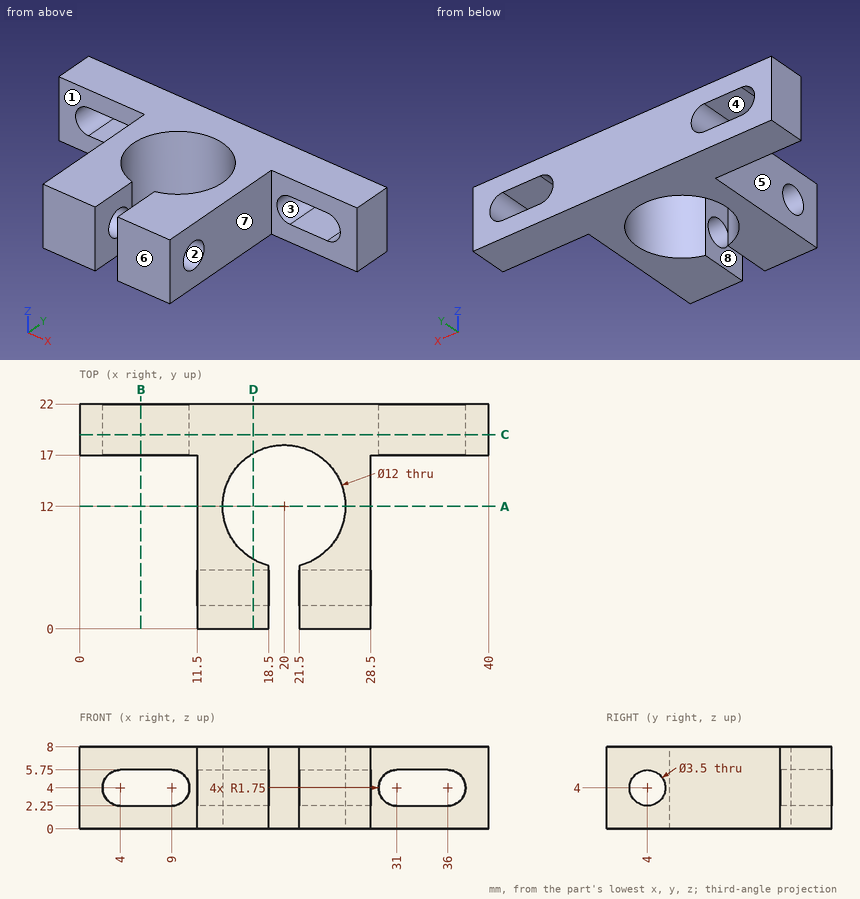
Geometry check sheet. Reference: drawing and pictorial views, mm from the part's lowest x, y, z. A direction names the side the tool comes from. Round coordinates to 2 decimals unless told otherwise and drop trailing zeros. Order: outer loops, then holes, each group sorted by start corner. A loop starts at its lowest first (then second) coordinate and runs counter-clockwise, first axis right, second up. Notation, with made-up numbers: (83.5, 75.25) - (112.5, 75.25) arc R25 ccw to (112.5, 111.25) - close; hole circle Ø2 at (88, -14.75). An arc over 180 degrees is marked (long way). Use a Markdown table: item, result. Add a question column.
1) Section check B-B (x = 6). Record the cut outline in (y, z).
2) Mould release check, pull along Y, two halves, no side actions. Record for the marked faces 1, 2 and 3: released by +Y, released by -Y, zero draft, split by the parting line, or undercut.
3) Thickness scan on line 1 along X through (y, z) = (4.5, 7.5); line 2 along Y through (x, z) = (16, 4.5); line 3 along Y through (x, z) = (25.25, 4). Record the ranges inside material, lowest first.
4) Gauge pin test, flat ends, axial feed: P1, Ø1, axis at x = 17, z = 4, coming from the -Y side; P2, Ø2.5, axis at y = 11.5, z = 4.5, coming from the -X side; P3, Ø4, axis at x = 35.5, z = 3.5, coming from the -Y side; P4, Ø4.5, axis at y = 4, z = 4, coming from the +X side. Record the tip position at first contact, or that the pin passes through.
5) Section check D-D (x = 17). Record the cut outline in (y, z).
6) Section check A-A (y = 12). Record the cut outline in (x, z).
7) Set-up check for the marked faces 4, 5, 6, 7 and 8: record each of +Z, -Z, +X, -X, +Y, -Y from which the full face is reachable in a straight line by a thin tool's end or side.
8) Section check C-C (y = 19). Record the cut outline in (x, z).
Established:
| question | item | result |
|---|---|---|
| 1 | outline | (17, 0) - (22, 0) - (22, 2.25) - (17, 2.25) - close; (17, 5.75) - (22, 5.75) - (22, 8) - (17, 8) - close |
| 2 | face 1 | released by -Y |
| 2 | face 2 | undercut |
| 2 | face 3 | zero draft |
| 3 | line 1 | 11.5 to 18.5, 21.5 to 28.5 |
| 3 | line 2 | 0 to 2.32, 5.68 to 7.53, 16.47 to 22 |
| 3 | line 3 | 0 to 2.25, 5.75 to 9.1, 14.9 to 22 |
| 4 | P1 | y = 0 |
| 4 | P2 | x = 11.5 |
| 4 | P3 | y = 17 |
| 4 | P4 | x = 28.5 |
| 5 | outline | (0, 0) - (6.8, 0) - (6.8, 8) - (0, 8) - close; (17.2, 0) - (22, 0) - (22, 8) - (17.2, 8) - close; hole circle Ø3.5 at (4, 4) |
| 6 | outline | (11.5, 0) - (14, 0) - (14, 8) - (11.5, 8) - close; (26, 0) - (28.5, 0) - (28.5, 8) - (26, 8) - close |
| 7 | face 4 | +Y, -Y |
| 7 | face 5 | +Z, -Z, -X, -Y |
| 7 | face 6 | +Z, -Z, +X, -X, -Y |
| 7 | face 7 | +Z, -Z, +X, -Y |
| 7 | face 8 | +Z, -Z, -Y |
| 8 | outline | (0, 0) - (40, 0) - (40, 8) - (0, 8) - close; hole (4, 2.25) - (9, 2.25) arc R1.75 ccw to (9, 5.75) - (4, 5.75) arc R1.75 ccw to start; hole (31, 2.25) - (36, 2.25) arc R1.75 ccw to (36, 5.75) - (31, 5.75) arc R1.75 ccw to start |
